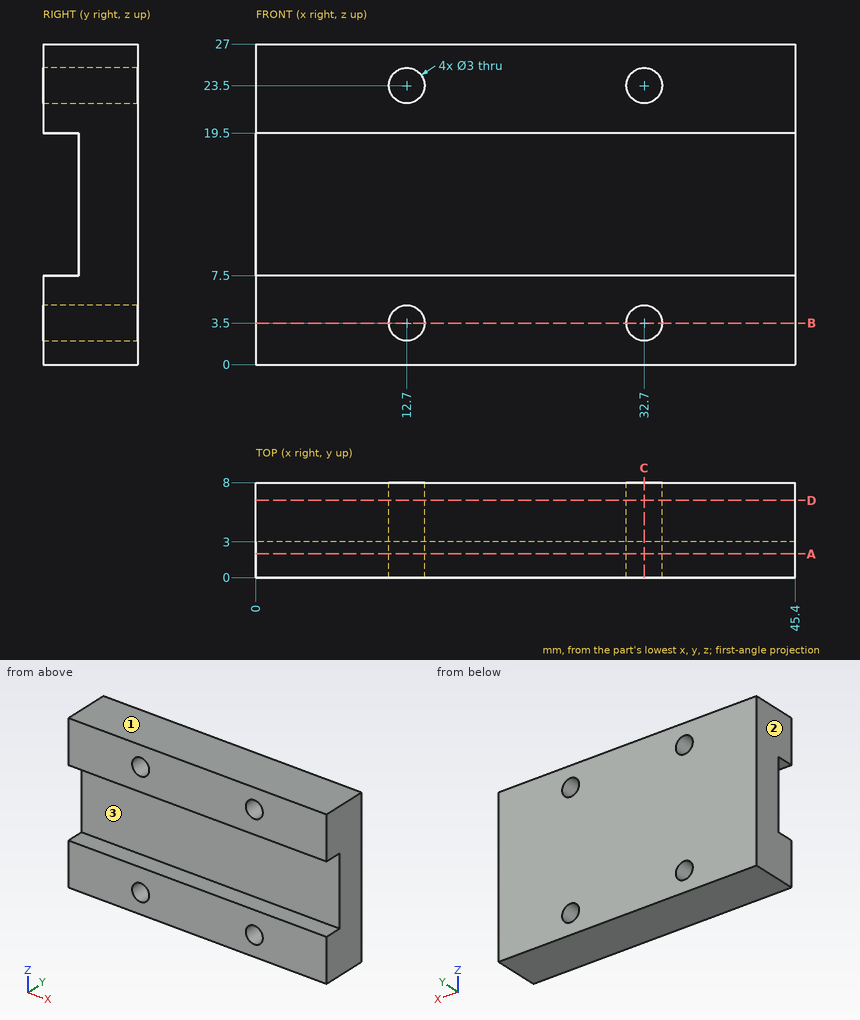
Input: dimensioned drawing with shaded views. Units: mm. Origin: part minimum x, y, z. Give positions to 0.01 mm unless a question says otherwise; leave off trailing zeros. Write each loop counter-clockwise with the first axis right and the second up, starting at its lowest first coordinate (ties: lowest second). Pieces come first, ordered by that corner, then holes. Notation, with made-up numbers: M 10,65.25 L 64,65.25 A34 cw 64,104.25 Z; hole C 62,-7 d9. An arc over 180 degrees is marked long. Return JSON: item names as keys, results as strings. Group by question number.
1) Pin query (flat end, axial travel): P1, Ø6, axis at x = 11.5, z = 15, coming from the -Y side. Return the tip coordinate at first contact, or that it passes through.
2) Cut plane D-D, the plane y = 6.5. Output: boundary loops of the cut face in (x, z).
3) Material intervals for line 1 along X through (y, z) = (4.5, 3.5); line 2 along Z through (x, y) = (32.7, 4.75); line 3 along Z through (x, y) = (31, 2), sorted ascending. Write a range as [from, to].
4) Cut plane C-C, the plane x = 32.7. Output: boundary loops of the cut face in (y, z).
5) Cut plane A-A, the plane y = 2. Output: boundary loops of the cut face in (x, z).
6) Cut plane B-B, the plane z = 3.5. Output: boundary loops of the cut face in (x, y), plus the area to 3 significant figures.
7) Pull-direction query (Z, two-part tool) for the marked faces 1, 2 and 3; classes: pulls with the +Z half, pulls with the -Z half, needs draft (parallel to the pull), parting line crosses it, or undercut.
Recorded:
{
 "1": {"P1": "stops at y = 3"},
 "2": {"outline": "M 0,0 L 45.4,0 L 45.4,27 L 0,27 Z; hole C 12.7,3.5 d3; hole C 12.7,23.5 d3; hole C 32.7,3.5 d3; hole C 32.7,23.5 d3"},
 "3": {"line 1": "x = [0, 11.2], [14.2, 31.2], [34.2, 45.4]", "line 2": "z = [0, 2], [5, 22], [25, 27]", "line 3": "z = [0, 7.5], [19.5, 27]"},
 "4": {"outline": "M 0,0 L 8,0 L 8,2 L 0,2 Z; M 0,5 L 8,5 L 8,22 L 0,22 L 0,19.5 L 3,19.5 L 3,7.5 L 0,7.5 Z; M 0,25 L 8,25 L 8,27 L 0,27 Z"},
 "5": {"outline": "M 0,0 L 45.4,0 L 45.4,7.5 L 0,7.5 Z; M 0,19.5 L 45.4,19.5 L 45.4,27 L 0,27 Z; hole C 12.7,3.5 d3; hole C 12.7,23.5 d3; hole C 32.7,3.5 d3; hole C 32.7,23.5 d3"},
 "6": {"outline": "M 0,0 L 11.2,0 L 11.2,8 L 0,8 Z; M 14.2,0 L 31.2,0 L 31.2,8 L 14.2,8 Z; M 34.2,0 L 45.4,0 L 45.4,8 L 34.2,8 Z", "area": "315 mm²"},
 "7": {"face 1": "pulls with the +Z half", "face 2": "needs draft", "face 3": "undercut"}
}
